Read the model definition and answer for the solid it produces. Units are mm, in the model's axes. Give positions to 0.01 mm unless a question says otherwise; leave off trailing zeros. Loops run counter-clockwise (first coordinate to the right, second up) from the corner with the lowest first, then second, coordinate; pieces in that order, holes last. Notation, with made-up numbers: (-38.5, 73.25) - (-1.5, 73.25) arc R27 ccw to (-1.5, 105.25) - close; hole circle Ø4 at (66, 7). An arc over 180 degrees is marked (long way). Write item = value, one per line.
Autodesk Inventor part; units mm, degrees
ref_plane "YZ Plane" through (0, 0, 0) normal (1, 0, 0) x (0, 1, 0)
ref_plane "XZ Plane" through (0, 0, 0) normal (0, 1, 0) x (-1, 0, 0)
ref_plane "XY Plane" through (0, 0, 0) normal (0, 0, 1) x (1, 0, 0)
sketch "Skizze2" plane through (0, 0, 0) normal (0, 0, 1) x (1, 0, 0)
  circle A0 centre (0, 0) radius 17.5
  circle A1 centre (0, 0) radius 19.5
  dimension "d0" = 35
  dimension "d1" = 39
extrude "Extrusion1" add sketch "Skizze2" along normal blind 30
sketch "Skizze3" plane through (0, 0, 0) normal (0, 0, -1) x (-1, 0, 0)
  circle A0 centre (0, 0) radius 17.5
extrude "Extrusion2" add sketch "Skizze3" against normal blind 20
fillet "Rundung1" radius 1 2 edges at (-17.5, 0, 30) (-19.5, 0, 30)
fillet "Rundung2" radius 1 1 edges at (-19.5, 0, 0)
properties part number "plug"
1) The mould has two halves that part along X. Classify faces 1 (the face through (0, 0, 20)), 2 (the face through (-2.539, -19.334, 14.804)), 3 (the face through (-13.887, 10.648, 24.437)), 4 (the face through (0, 0, 0)): pulls with the +X half, pulls with the -X half, needs draft (parallel to the pull), parting line crosses it, or undercut.
Output:
face_1 = undercut
face_2 = parting line crosses it
face_3 = undercut
face_4 = needs draft
2) Find the intervals of material crossed by probe 1 along Y at (x, z) = (0, 24.75); probe 2 along Z at (x, y) = (-1.5, -1); probe 3 along Y at (x, z) = (-6.5, 26.5), in increasing order.
Output:
probe_1 = -19.5 to -17.5, 17.5 to 19.5
probe_2 = 0 to 20
probe_3 = -18.38 to -16.25, 16.25 to 18.38
3) A cutting plane is placed at C-C on z = 24. Determine the outline of the cut face in (x, y), then the cut area to 3 significant figures.
Output:
outline = circle Ø39 at (0, 0); hole circle Ø35 at (0, 0)
area = 232 mm²
4) Each of these flat-tipped pins is pushed along its axis until it touches: P1, Ø6, axis at y = 3.5, z = 27, coming from the +X side; P2, Ø12, axis at x = 13.5, y = -15, coming from the -Z side; P3, Ø2, axis at y = 7, z = 14.5, coming from the +X side; P4, Ø12, axis at y = 13, z = 21, coming from the -X side. Where does it stop, or does it pass through?
Output:
P1 = 19.49
P2 = 0
P3 = 18.55
P4 = -18.2
5) A cutting plane is placed at D-D on z = 9. Determine the outline of the cut face in (x, y).
Output:
outline = circle Ø39 at (0, 0)
